Work out the finished part from the listing and answer in its coordinate system (mm). Round coordinates to 2 decimals unless told otherwise and drop trailing zeros. Write each loop counter-clockwise with the first axis right and the second up, starting at its lowest first coordinate (ties: lowest second). Pieces come first, ordered by that corner, then holes. Notation, with made-up numbers: (84, 62.25) -> (96, 62.25) arc R9 cw to (96, 78.25) -> close; hole circle Ø6 at (50, -18). An arc over 180 degrees is marked (long way). Answer as a JSON object with one key per item and string values. Group by question number.
from build123d import *

# Parameters (mm, degrees)
EXTRUDE_1_DEPTH = 20
SKETCH_2_R      = 30
EXTRUDE_2_DEPTH = 35


with BuildPart() as part:
    # 草图1 → 凸台-拉伸1 (new body)
    with BuildSketch(Plane(origin=(0, 0, 0), x_dir=(0, 0, -1), z_dir=(1, 0, 0))):
        with BuildLine():
            Line((0, 30), (-200, 30))
            ThreePointArc((-200, 30), (-230, 0), (-200, -30))
            Line((-200, -30), (0, -30))
            ThreePointArc((0, -30), (30, 0), (0, 30))
        make_face()
    extrude(amount=EXTRUDE_1_DEPTH)

    # 草图2 → 凸台-拉伸2 (add)
    with BuildSketch(Plane.ZY):
        Circle(SKETCH_2_R)
    extrude(amount=EXTRUDE_2_DEPTH)


solid = part.part
1) A cutting plane is placed at A-A on y = -18. Determine the outline of the cut face in (x, z), plus the area to 3 significant figures.
2) A cutting plane is placed at B-B on x = -8. Determine the outline of the cut face in (y, z).
3) A cutting plane is placed at D-D on y = 0. Determine the outline of the cut face in (x, z), plus the area to 3 significant figures.
4) Each of these flat-tipped pins is pushed along its axis until it touches: P1, Ø3, axis at y = -10.5, z = 30.5, coming from the -X side; P2, Ø5, axis at x = -19.5, y = 6, coming from the +Z side. Where does it stop, or does it pass through?
5) For a pull along Z with two mould halves and no side action, classify faces 1 (the face through (9.86, 0.66, 229.993)), 2 (the face through (-35, 0, 0)) as released by +Z, released by -Z, zero draft, split by the parting line, or undercut.
6) Straight lines are drawn through the part: L1, parallel to X at y = 1, z = 165; L2, parallel to Z at x = -31, y = 7.5; L3, parallel to Z at x = -20.5, y = 4.5. For each, find the intervals that lie inside material, in ascending order.
7) A cutting plane is placed at C-C on z = 98. Determine the outline of the cut face in (x, y), plus the area to 3 significant figures.
Established:
{
 "1": {"outline": "(-35, -24) -> (20, -24) -> (20, 224) -> (0, 224) -> (0, 24) -> (-35, 24) -> close", "area": "6,640 mm²"},
 "2": {"outline": "circle Ø60 at (0, 0)"},
 "3": {"outline": "(-35, -30) -> (20, -30) -> (20, 230) -> (0, 230) -> (0, 30) -> (-35, 30) -> close", "area": "7,300 mm²"},
 "4": {"P1": "stops at x = 0", "P2": "stops at z = 29.8"},
 "5": {"face 1": "released by +Z", "face 2": "zero draft"},
 "6": {"L1": "x = 0 to 20", "L2": "z = -29.05 to 29.05", "L3": "z = -29.66 to 29.66"},
 "7": {"outline": "(0, -30) -> (20, -30) -> (20, 30) -> (0, 30) -> close", "area": "1,200 mm²"}
}
